Design review of the part shown in the three views and the two pictorial views. Dimensions are in mm from the part's minimum x, y and z. Coordinates: 2 decimals unless noted, no trailing zeros. Order: outer loops, then holes, each group sorted by start corner. A loop starts at its lowest first (then second) coordinate and runs counter-clockwise, first axis right, second up. Notation, with made-up numbers: (53.25, 82.5) -> (59.25, 82.5) arc R12 ccw to (59.25, 86.5) -> close; hole circle Ø5 at (-39.75, -8.5). An arc over 180 degrees is marked (long way). Answer as a JSON object with one key per item and string values. Group by question number.
1) For pin 1 (20.5 mm diameter, centred on y = 1129.5, z = 32, fed in from -X); pin 2 (10 mm diameter, centred on x = 330.2, y = 1181.1, fed in from +Z) (3 decimals); pin 3 (20.5 mm diameter, centred on y = 1161.5, z = 191, fed in from +X), all flat-tipped, find the tip position at first contact; note any pin that passes through.
2) Add section C-C, the plane y = 604. Write out the cut boundary in (x, z).
3) Add section B-B, the plane z = 27.5. Write out the cut boundary in (x, y), then the cut area to 3 significant figures.
4) Add section D-D, the plane x = 199. Write out the cut boundary in (y, z), then the cut area to 3 significant figures.
5) Add section A-A, the plane x = 393.5. Write out the cut boundary in (y, z).
6) Wall thickness on L1, parallel to X at y = 1181.1, z = 16; L2, parallel to Y at x = 330, z = 24; L3, parallel to X at y = 942, z = 31.5: over which ranges is each line inside the solid? List them lowest first.
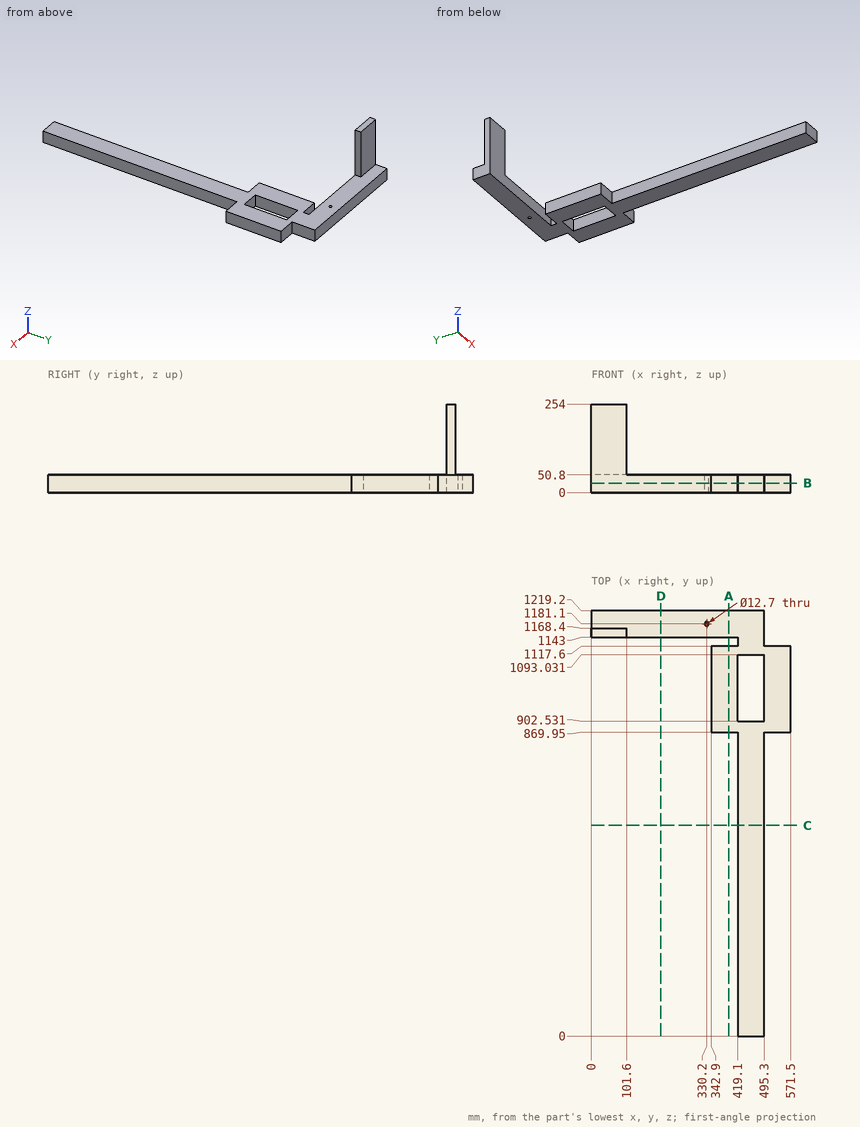
Output values:
{
 "1": {"pin 1": "stops at x = 419.1", "pin 2": "passes through", "pin 3": "stops at x = 101.6"},
 "2": {"outline": "(419.1, 0) -> (495.3, 0) -> (495.3, 50.8) -> (419.1, 50.8) -> close"},
 "3": {"outline": "(0, 1143) -> (419.1, 1143) -> (419.1, 1117.6) -> (342.9, 1117.6) -> (342.9, 869.95) -> (419.1, 869.95) -> (419.1, 0) -> (495.3, 0) -> (495.3, 869.95) -> (571.5, 869.95) -> (571.5, 1117.6) -> (495.3, 1117.6) -> (495.3, 1219.2) -> (0, 1219.2) -> close; hole circle Ø12.7 at (330.2, 1181.1); hole (419.1, 902.53) -> (495.3, 902.53) -> (495.3, 1093.03) -> (419.1, 1093.03) -> close", "area": "148,000 mm²"},
 "4": {"outline": "(1143, 0) -> (1219.2, 0) -> (1219.2, 50.8) -> (1143, 50.8) -> close", "area": "3,870 mm²"},
 "5": {"outline": "(869.95, 0) -> (1117.6, 0) -> (1117.6, 50.8) -> (869.95, 50.8) -> close; (1143, 0) -> (1219.2, 0) -> (1219.2, 50.8) -> (1143, 50.8) -> close"},
 "6": {"L1": "x = 0 to 323.85, 336.55 to 495.3", "L2": "y = 1143 to 1174.75, 1187.45 to 1219.2", "L3": "x = 342.9 to 419.1, 495.3 to 571.5"}
}
